Could you check a few things on this model? Use its own coordinates, in mm. A direction names the side the tool comes from. Round coordinates to 2 decimals unless told otherwise and drop trailing zeros. Write each loop counter-clockwise with the first axis right and the second up, starting at its lowest first coordinate (ties: lowest second). Pieces come first, ordered by that corner, then holes. Notation, with made-up numbers: (89.5, -9) -> (124.5, -9) arc R6 ccw to (124.5, -5) -> close; hole circle Ø9 at (61, 38). An arc over 180 degrees is marked (long way). Answer as CSV lines item,"result". Start each with the question number.
Q1. Will this pin go through, and if not, where does the flat tip stop? pin 1 Ø4 at (x, z) = (-38.5, 31) entering from -Y.
Q2. If we mould it in two halves opening along X, with no side actions, what happens to faces 3 (the flat face through (90, 151, 89)), 4 (the flat face through (-90, 89, 29)), 5 (the flat face through (-1, 180, 49)), 6 (the cylindrical face through (1.32, 176.06, 60.03))? For each: pulls with the +X half, pulls with the -X half, needs draft (parallel to the pull), parting line crosses it, or undercut.
Q3. If I drill on line 1 (Z direction, x = 85, y = 90); line 2 (X direction, y = 29.5, z = 151); line 3 (X direction, y = 175.5, z = 90), over which ranges is the centre line in solid material (lowest first)? Write a range as [from, to].
Q4. For faces 1 (the flat face through (0, 177, 0)), 2 (the flat face through (38, 172, 89)), which set-ups out of +Z, -Z, +X, -X, +Y, -Y let a thin tool reach every point of the face, with its end or its side?
Q5. Imagine slicing it at C-C on y = 12. Please give me the cut outline in (x, z).
Q6. Imagine slicing it at D-D on z = 38.5. Please give me the cut outline in (x, y), and give its area (3 significant figures).
Q7. Imagine slicing it at B-B on x = 0. Please give me the cut outline in (y, z).
Q8. Imagine slicing it at A-A on y = 90. Please give me the cut outline in (x, z), and give its area (3 significant figures).
from build123d import *

# Parameters (mm, degrees)
EXTRUDE_1_DEPTH     = 180
SKETCH_2_R          = 30
CUT_EXTRUDE_1_DEPTH = 180
SKETCH_3_R          = 60
CUT_EXTRUDE_2_DEPTH = 217


with BuildPart() as part:
    # 草图1 → 凸台-拉伸1 (new body)
    with BuildSketch(Plane.XY):
        Polygon((-90, 180), (90, 180), (90, 0), (82, 0), (82, 172), (-82, 172), (-82, 0), (-90, 0), align=None)
    extrude(amount=EXTRUDE_1_DEPTH)

    # 草图2 → 切除-拉伸1 (cut)
    with BuildSketch(Plane(origin=(0, 180, 0), x_dir=(1, 0, 0), z_dir=(0, 1, 0))):
        with Locations(Location((0, -90, 0), (0, 0, 270))):
            Circle(SKETCH_2_R)
    extrude(amount=-CUT_EXTRUDE_1_DEPTH, mode=Mode.SUBTRACT)

    # 草图3 → 切除-拉伸2 (cut)
    with BuildSketch(Plane(origin=(90, 0, 0), x_dir=(0, 0, -1), z_dir=(1, 0, 0))):
        with Locations(Location((-90, 90, 0), (0, 0, 90))):
            Circle(SKETCH_3_R)
    extrude(amount=-CUT_EXTRUDE_2_DEPTH, mode=Mode.SUBTRACT)


solid = part.part
Checks:
1,pin 1,"y = 172"
2,face 3,"pulls with the +X half"
2,face 4,"pulls with the -X half"
2,face 5,"needs draft"
2,face 6,"undercut"
3,line 1,"[0, 30], [150, 180]"
3,line 2,"[-90, -82], [82, 90]"
3,line 3,"[-90, -30], [30, 90]"
4,face 1,"-Z, +X, -X, +Y, -Y"
4,face 2,"+Z, -Z, -Y"
5,outline,"(-90, 0) -> (-82, 0) -> (-82, 180) -> (-90, 180) -> close; (82, 0) -> (90, 0) -> (90, 180) -> (82, 180) -> close"
6,outline,"(-90, 0) -> (-82, 0) -> (-82, 59.21) -> (-90, 59.21) -> close; (-90, 120.79) -> (-82, 120.79) -> (-82, 172) -> (82, 172) -> (82, 120.79) -> (90, 120.79) -> (90, 180) -> (-90, 180) -> close; (82, 0) -> (90, 0) -> (90, 59.21) -> (82, 59.21) -> close"
6,area,"3,210 mm^2"
7,outline,"(172, 0) -> (180, 0) -> (180, 60) -> (172, 60) -> close; (172, 120) -> (180, 120) -> (180, 180) -> (172, 180) -> close"
8,outline,"(-90, 0) -> (-82, 0) -> (-82, 30) -> (-90, 30) -> close; (-90, 150) -> (-82, 150) -> (-82, 180) -> (-90, 180) -> close; (82, 0) -> (90, 0) -> (90, 30) -> (82, 30) -> close; (82, 150) -> (90, 150) -> (90, 180) -> (82, 180) -> close"
8,area,"960 mm^2"
